Verification items for the finished model (mm, model axes). A direction names the side the tool comes from. Round coordinates to 2 decimals unless told otherwise and drop trailing zeros. Write each loop counter-clockwise with the first axis right and the second up, starting at its lowest first coordinate (ties: lowest second). Pieces come first, ordered by that corner, then holes. Notation, with made-up numbers: M 80.25,9.25 L 110.25,9.25 A16 cw 110.25,15.25 Z; hole C 30.5,-21.5 d10. An arc over 180 degrees is marked long. Answer in a Markdown table with one row per item. Add a question column.
1. Go/stop test with flat-tipped pins: pin 1 Ø2 at (x, y) = (-9.525, -2) entering from +Z; pin 2 Ø11 at (x, y) = (0, -2) entering from +Z; pin 3 Ø1.5 at (y, z) = (6.5, 5) entering from -X; pin 4 Ø5 at (x, y) = (19.5, 4) entering from +Z. Record where each tip stops, or that it passes through.
2. Sectioned sample at A-A on z = 18.25. Record the cut outline in (x, y).
3. Sectioned sample at D-D on y = -2. Count the separate pieces of the cut face and the enclosed holes in it, plus the area to 3 significant figures.
4. Sectioned sample at C-C on z = 9. Record the cut outline in (x, y) (3 decimals).
5. Sectioned sample at B-B on x = 0. Record the cut outline in (y, z).
6. Set-up check for faces 4 (the cylindrical face through (-20.69, 0.63, 23.27)), 5 (the flat face through (6, -5, 3)), 6 (the flat face through (0, 5, 16.15)), 7 (the cylindrical face through (23.1, -0.14, 9.14)): record each of +Z, -Z, +X, -X, +Y, -Y from which the full face is reachable in a straight line by a thin tool's end or side.
7. Material ranges on probe 1 along Y at (x, z) = (0, 13.7); probe 2 along Y at (x, z) = (0, 3.25); probe 3 along Z at (x, y) = (-22, -1), recorded low to high.
8. Draft check along Y on faces 1 (the flat face through (30.125, 0, 13)), 2 (the flat face through (6, -5, 11)), 3 (the flat face through (23.8, -9, 21.5)). Enter one of: pulls with the +Y half, pulls with the -Y half, needs draft (parallel to the pull), parting line crosses it, or undercut.
```python
from build123d import *

# Parameters (mm, degrees)
ESQUISSE2_W                         = 60.25
ESQUISSE2_H                         = 20
BOSS_EXTRU_2_DEPTH                  = 25.15
ESQUISSE3_W                         = 29.75
ESQUISSE3_H                         = 20
ENL_V_MAT_EXTRU_1_DEPTH             = 9
ESQUISSE4_W                         = 48
ESQUISSE4_H                         = 6
ENL_V_MAT_EXTRU_2_DEPTH             = 45.045863881
ESQUISSE5_R                         = 6
ENL_V_MAT_EXTRU_3_DEPTH             = 36.613735061
ENL_V_START                         = -1
ESQUISSE6_R                         = 7
ENL_V_MAT_EXTRU_4_DEPTH             = 8
ESQUISSE7_R                         = 6.025
ENL_V_MAT_EXTRU_5_DEPTH             = 45.045863881
CONG_1_R                            = 7.5
CONG_2_R                            = 0.5
DIAM_TRE_DU_PER_AGE_2_5_2_5_1_D     = 2.5
DIAM_TRE_DU_PER_AGE_2_5_2_5_1_DEPTH = 6.15
CONG_4_R                            = 3
BOSS_EXTRU_3_START                  = -1
ESQUISSE11_R                        = 6.025
ESQUISSE11_R_2                      = 4
BOSS_EXTRU_3_DEPTH                  = 1
CHANFREIN2_SIZE                     = 0.3


with BuildPart() as part:
    # Esquisse2 → Boss.-Extru.2 (new body)
    with BuildSketch(Plane.XY):
        Rectangle(ESQUISSE2_W, ESQUISSE2_H)
    extrude(amount=BOSS_EXTRU_2_DEPTH)

    # Esquisse3 → Enlèv. mat.-Extru.1 (cut)
    with BuildSketch(Plane.XY.offset(25.15)):
        Rectangle(ESQUISSE3_W, ESQUISSE3_H)
    extrude(amount=-ENL_V_MAT_EXTRU_1_DEPTH, mode=Mode.SUBTRACT)

    # Esquisse4 → Enlèv. mat.-Extru.2 (cut, through all)
    with BuildSketch(Plane(origin=(0, 10, 0), x_dir=(1, 0, 0), z_dir=(0, 1, 0))):
        with Locations((0, -7)):
            Rectangle(ESQUISSE4_W, ESQUISSE4_H)
    extrude(amount=-ENL_V_MAT_EXTRU_2_DEPTH, mode=Mode.SUBTRACT)

    # Esquisse5 → Enlèv. mat.-Extru.3 (cut, through all)
    with BuildSketch(Plane.XY.offset(16.15)):
        with Locations((0, -2)):
            Circle(ESQUISSE5_R)
    extrude(amount=-ENL_V_MAT_EXTRU_3_DEPTH, mode=Mode.SUBTRACT)

    # Esquisse6 → Enlèv. mat.-Extru.4 (cut)
    with BuildSketch(Plane.XY.offset(4).offset(ENL_V_START)):
        with Locations(Location((0, -2, 0), (0, 0, 180))):
            Circle(ESQUISSE6_R)
    extrude(amount=ENL_V_MAT_EXTRU_4_DEPTH, mode=Mode.SUBTRACT)

    # Esquisse7 → Enlèv. mat.-Extru.5 (cut, through all)
    with BuildSketch(Plane(origin=(0, 10, 0), x_dir=(1, 0, 0), z_dir=(0, 1, 0))):
        with Locations(Location((-22.5, -17.525, 0), (0, 0, 270))):
            Circle(ESQUISSE7_R)
        with Locations(Location((22.5, -17.525, 0), (0, 0, 270))):
            Circle(ESQUISSE7_R)
    extrude(amount=-ENL_V_MAT_EXTRU_5_DEPTH, mode=Mode.SUBTRACT)

    # Congé1
    cong_1_edges = [part.edges().sort_by_distance(p)[0] for p in [
        (-30.125, 0, 25.15),
        (14.875, 0, 25.15),
        (-14.875, 0, 25.15),
        (-30.125, 0, 0),
        (30.125, 0, 0),
        (30.125, 0, 25.15),
    ]]
    fillet(cong_1_edges, radius=CONG_1_R)

    # Congé2
    cong_2_edges = [part.edges().sort_by_distance(p)[0] for p in [
        (14.875, 0, 16.15),
        (-14.875, 0, 16.15),
    ]]
    fillet(cong_2_edges, radius=CONG_2_R)

    # Diamètre du perçage Ø2.5 (2.5)1
    with Locations(Plane.XY.offset(16.15)):
        with Locations((-9.525, -2), (9.525, -2)):
            Hole(DIAM_TRE_DU_PER_AGE_2_5_2_5_1_D / 2, depth=DIAM_TRE_DU_PER_AGE_2_5_2_5_1_DEPTH)

    # Congé4
    cong_4_edges = [part.edges().sort_by_distance(p)[0] for p in [
        (-24, 0, 10),
        (-24, 0, 4),
        (24, 0, 4),
        (24, 0, 10),
    ]]
    fillet(cong_4_edges, radius=CONG_4_R - 0.0001)  # a hair under: the kernel refuses the full size

    # Esquisse11 → Boss.-Extru.3 (add)
    # profile 1 of 2: a face of its own
    with BuildSketch(Plane.XZ.offset(10).offset(BOSS_EXTRU_3_START)):
        with Locations(Location((22.5, 17.525, 0), (0, 0, 90))):
            Circle(ESQUISSE11_R)
        with Locations(Location((22.5, 17.525, 0), (0, 0, 270))):
            Circle(ESQUISSE11_R_2, mode=Mode.SUBTRACT)
    # profile 2 of 2: a face of its own
    with BuildSketch(Plane.XZ.offset(10).offset(BOSS_EXTRU_3_START)):
        with Locations(Location((-22.5, 17.525, 0), (0, 0, 90))):
            Circle(ESQUISSE11_R)
        with Locations(Location((-22.5, 17.525, 0), (0, 0, 270))):
            Circle(ESQUISSE11_R_2, mode=Mode.SUBTRACT)
    extrude(amount=BOSS_EXTRU_3_DEPTH)

    # Chanfrein2
    chanfrein2_edges = [part.edges().sort_by_distance(p)[0] for p in [
        (-6, -2, 11),
        (-6, -2, 3),
    ]]
    chamfer(chanfrein2_edges, length=CHANFREIN2_SIZE)


solid = part.part
```
Geometry check:
| question | item | result |
|---|---|---|
| 1 | pin 1 | stops at z = 4 |
| 1 | pin 2 | passes through |
| 1 | pin 3 | stops at x = -29.92 |
| 1 | pin 4 | stops at z = 25.14 |
| 2 | outline | M -30.1,-10 L -26.43,-10 L -26.43,-9 L -28.48,-9 L -28.48,10 L -30.1,10 Z; M -18.57,-10 L -14.9,-10 L -14.9,10 L -16.52,10 L -16.52,-9 L -18.57,-9 Z; M 14.9,-10 L 18.57,-10 L 18.57,-9 L 16.52,-9 L 16.52,10 L 14.9,10 Z; M 26.43,-10 L 30.1,-10 L 30.1,10 L 28.48,10 L 28.48,-9 L 26.43,-9 Z |
| 3 | separate pieces | 4 |
| 3 | enclosed holes | 2 |
| 3 | area | 510 mm2 |
| 4 | outline | M -30.125,-10 L -23.236,-10 L -23.236,10 L -30.125,10 Z; M 23.236,-10 L 30.125,-10 L 30.125,10 L 23.236,10 Z |
| 5 | outline | M -10,0 L -8,0 L -8,2.7 L -8.3,3 L -9,3 L -9,4 L -10,4 Z; M -10,10 L -9,10 L -9,11 L -8.3,11 L -8,11.3 L -8,16.15 L -10,16.15 Z; M 4,0 L 10,0 L 10,4 L 5,4 L 5,3 L 4.3,3 L 4,2.7 Z; M 4,11.3 L 4.3,11 L 5,11 L 5,10 L 10,10 L 10,16.15 L 4,16.15 Z |
| 6 | face 4 | +Y |
| 6 | face 5 | none |
| 6 | face 6 | +Z, +Y, -Y |
| 6 | face 7 | +Y, -Y |
| 7 | probe 1 | y = -10 to -8, 4 to 10 |
| 7 | probe 2 | y = -10 to -9, 5 to 10 |
| 7 | probe 3 | z = 0 to 4.17, 9.83 to 11.52, 23.53 to 25.14 |
| 8 | face 1 | needs draft |
| 8 | face 2 | undercut |
| 8 | face 3 | pulls with the +Y half |
